```python
from build123d import *

# Parameters (mm, degrees)
F1_DEPTH = 63.5
F2_DEPTH = 25.4
F3_DEPTH = 7.9375
F0_W     = 25.4
F0_H     = 19.0500000358
F4_DEPTH = 25.4
F6_R     = 6.35


with BuildPart() as f1:
    # F0 (on Front) → F1 (new body, symmetric)
    with BuildSketch(Plane.XZ):
        Polygon((41.275, -9.525), (41.275, 9.525), (22.2249999642, 9.525), (-41.275, 9.525), (-41.275, -9.525), align=None)
    extrude(amount=F1_DEPTH, both=True)

    # F0 (on Front) → F2 (join, symmetric)
    with BuildSketch(Plane.XZ):
        with BuildLine():
            Line((22.2249999642, 9.525), (41.275, 9.525))
            Line((41.275, 9.525), (41.275, 27.0002))
            ThreePointArc((41.275, 27.0002), (45.9246798487, 38.2255201513), (57.15, 42.8752))
            Line((57.15, 42.8752), (60.325, 42.8752))
            Line((60.325, 42.8752), (60.325, 61.9252000358))
            Line((60.325, 61.9252000358), (57.15, 61.9252000358))
            add(Edge.make_bspline(
                [(54.2137588314, 61.801552205), (55.2005191802, 61.8492221851), (56.1795792911, 61.8903742324), (57.15, 61.9252000358)],
                knots=[108.8573598522, 108.8573598522, 108.8573598522, 108.8573598522, 111.5045361803, 111.5045361803, 111.5045361803, 111.5045361803], degree=3))
            ThreePointArc((54.2137588314, 61.801552205), (31.4371253025, 50.6349985456), (22.2249999642, 27.0002))
            Line((22.2249999642, 27.0002), (22.2249999642, 9.525))
        make_face()
    extrude(amount=F2_DEPTH, both=True)

    # F0 (on Front) → F3 (join, symmetric)
    with BuildSketch(Plane.XZ):
        with BuildLine():
            Line((-41.275, 9.525), (22.2249999642, 9.525))
            Line((22.2249999642, 9.525), (22.2249999642, 27.0002))
            ThreePointArc((22.2249999642, 27.0002), (31.4371253025, 50.6349985456), (54.2137588314, 61.801552205))
            add(Edge.make_bspline(
                [(-41.275, 9.525), (-39.9627792732, 46.8589932408), (13.6361345752, 59.8412641353), (54.2137588314, 61.801552205)],
                knots=[0, 0, 0, 0, 108.8573598522, 108.8573598522, 108.8573598522, 108.8573598522], degree=3))
        make_face()
    extrude(amount=F3_DEPTH, both=True)

    # F0 (on Front) → F4 (join, symmetric)
    with BuildSketch(Plane.XZ):
        with Locations((73.025, 52.4002000179)):
            Rectangle(F0_W, F0_H)
    extrude(amount=F4_DEPTH, both=True)

    # F0 (on Front) → F5 (revolve)
    with BuildSketch(Plane.XZ):
        Polygon((85.725, 61.9252000358), (85.725, 42.8752), (85.725, 38.1), (111.125, 38.1), (111.125, 66.675), (85.725, 66.675), align=None)
    revolve(axis=Axis((85.725, 0, 52.3875), (0, 0, 1)))

    # F6
    f6_edges = [f1.edges().sort_by_distance(p)[0] for p in [
        (41.275, -63.5, 0),
        (-41.275, -63.5, 0),
        (-41.275, 63.5, 0),
        (41.275, 63.5, 0),
    ]]
    fillet(f6_edges, radius=F6_R)


solid = f1.part
```
Part model, mm, in its own coordinate system. A direction names the side the tool comes from. Coordinates: 2 decimals unless noted, no trailing zeros. Order: outer loops, then holes, each group sorted by start corner. A loop starts at its lowest first (then second) coordinate and runs counter-clockwise, first axis right, second up. Notation, with made-up numbers: (21.5, -6) - (32.5, -6) arc R28 cw to (32.5, 23) - close; hole circle Ø3 at (51.25, 11.5). An arc over 180 degrees is marked (long way). Return JSON: item names as keys, results as strings. Group by question number.
Item 1: Which spindle directions (+Z, -Z, +X, -X, +Y, -Y) get a long thin tool onto all of the face, cutting with end or side? Do faces 1 (the face through (-5, -7.938, 30)), 2 (the face through (31.684, 16.547, 50.901)), 3 (the face through (46, 25.4, 42)), 4 (the face through (86, 0, 38.1)). Say none if no direction does.
Item 2: Pin check, flat tips, straight feed: pin 1 (16.5 mm diameter, centred on x = 17.5, y = 37, fed in from +Z) (3 decimals); pin 2 (11 mm diameter, centred on y = -5.5, z = 6.5, fed in from +X) (3 decimals); pin 3 (2 mm diameter, centred on x = 85, y = -13, fed in from -Z). Stop position of each tip, or through.
Item 3: Cut at B-B (y = 32.5). List the corners of the cut face in (x, z) (3 decimals), plus the area to 3 significant figures.
Item 4: Cut at A-A (x = 68.5). List the corners of the cut face in (y, z) (3 decimals).
Item 5: Drill centre lines: probe 1 along Z at (x, y) = (38, -34) (3 decimals); probe 2 along Z at (x, y) = (75.5, 0) (3 decimals); probe 3 along Y at (x, z) = (19, 45). Where is each one in solid material? Low to high. Write a range as from..to.
Check values:
{
 "1": {"face 1": "+Z, -X, -Y", "face 2": "+Z, -X, +Y", "face 3": "+Z, +X, -X, +Y", "face 4": "-Z, +X, +Y, -Y"},
 "2": {"pin 1": "stops at z = 9.525", "pin 2": "stops at x = 41.275", "pin 3": "stops at z = 38.1"},
 "3": {"outline": "(-41.275, -9.525) - (41.275, -9.525) - (41.275, 9.525) - (-41.275, 9.525) - close", "area": "1,570 mm2"},
 "4": {"outline": "(-25.4, 42.875) - (-18.667, 42.875) - (-18.667, 38.1) - (18.667, 38.1) - (18.667, 42.875) - (25.4, 42.875) - (25.4, 61.925) - (18.667, 61.925) - (18.667, 66.675) - (-18.667, 66.675) - (-18.667, 61.925) - (-25.4, 61.925) - close"},
 "5": {"probe 1": "z = -9.525..9.525", "probe 2": "z = 38.1..66.675", "probe 3": "y = -7.94..7.94"}
}
